Design review of the part built by this model. Coordinates are the model's own, in mm. Face numbers are marked on the shaded views. A direction names the side the tool comes from. Round coordinates to 2 decimals unless told otherwise and drop trailing zeros. Loops run counter-clockwise (first coordinate to the right, second up) from the corner with the lowest first, then second, coordinate; pieces in that order, holes last. Notation, with made-up numbers: (25, 48.5) -> (77, 48.5) arc R33 cw to (77, 79.5) -> close; hole circle Ø5 at (0, 40.25). An arc over 180 degrees is marked (long way). Answer as CSV lines item,"result". Start each with the question number.
(1) Take a section at C-C, the plane y = -3.25. Write out the cut boundary in (x, z), and give its area (3 significant figures).
(2) Draft analysis for pull direction Y (two halves, no side actions). For the marked faces 5, 6, 7 and 8, state which applies: +Y half, -Y half, draft (parallel to the pull), parting line (faces both ways), or undercut.
(3) Take a section at A-A, the plane x = 0. Write out the cut boundary in (y, z).
(4) Take a section at D-D, the plane x = -3.25. Write out the cut boundary in (y, z).
(5) Take a section at B-B, the plane z = 8.5. Write out the cut boundary in (x, y), and give its area (3 significant figures).
(6) Machinability: for the marked faces 1, 2, 3 and 4, which of the approach directions +Z, -Z, +X, -X, +Y, -Y give a long, thin tool a straight path to every point of the face, cutting with its end or side? Answer none if there is none.
(7) For P1, Ø1, axis at x = 6, z = 9.5, coming from the +Y side; P2, Ø0.6, axis at y = 8.5, z = 1.5, coming from the +X side; P3, Ø0.6, axis at y = 8.5, z = 1, coming from the -X side, all flat-tipped, find the tip position at first contact; note any pin that passes through.
(8) To check wall thickness, follow line 1 (Y direction, x = 0, z = 1.1); line 2 (Y direction, x = 0, z = 0.65); line 3 (Z direction, x = 1.5, y = -1.25). State the ranges of each line that lie inside material, in increasing order. Write a range as from..to.
from build123d import *

# Parameters (mm, degrees)
SKETCH1_W           = 20
SKETCH1_H           = 14
BOSS_EXTRUDE1_DEPTH = 12
SKETCH2_R           = 1.5
BOSS_EXTRUDE2_DEPTH = 2
SHELL2_START        = -6
SHELL2_OUTLINE_W    = 20
SHELL2_OUTLINE_H    = 10
SHELL2_DEPTH        = 12


# Read off the part's stored shape, not the designer's step: Shell2
with BuildPart() as part:
    # Sketch1 → Boss-Extrude1 (new body)
    with BuildSketch(Plane.XY):
        Rectangle(SKETCH1_W, SKETCH1_H)
    extrude(amount=BOSS_EXTRUDE1_DEPTH)

    # Sketch2 → Boss-Extrude2 (add)
    # profile 1 of 2: a face of its own
    with BuildSketch(Plane.XY):
        with BuildLine():
            Line((2.5, -9.5), (2.5, -7))
            Line((2.5, -7), (-2.5, -7))
            Line((-2.5, -7), (-2.5, -9.5))
            ThreePointArc((-2.5, -9.5), (0, -12), (2.5, -9.5))
        make_face()
        with Locations((0, -9.5)):
            Circle(SKETCH2_R, mode=Mode.SUBTRACT)
    # profile 2 of 2: a face of its own
    with BuildSketch(Plane.XY):
        with BuildLine():
            Line((2.5, 9.5), (2.5, 7))
            Line((2.5, 7), (-2.5, 7))
            Line((-2.5, 7), (-2.5, 9.5))
            ThreePointArc((-2.5, 9.5), (0, 12), (2.5, 9.5))
        make_face()
        with Locations((0, 9.5)):
            Circle(SKETCH2_R, mode=Mode.SUBTRACT)
    extrude(amount=BOSS_EXTRUDE2_DEPTH)

    # Shell2 outline → Shell2 (cut)
    with BuildSketch(Plane(origin=(0, 0, 0), x_dir=(1, 0, 0), z_dir=(0, 1, 0)).offset(SHELL2_START)):
        with Locations((0, -6)):
            Rectangle(SHELL2_OUTLINE_W, SHELL2_OUTLINE_H)
    extrude(amount=SHELL2_DEPTH, mode=Mode.SUBTRACT)


solid = part.part
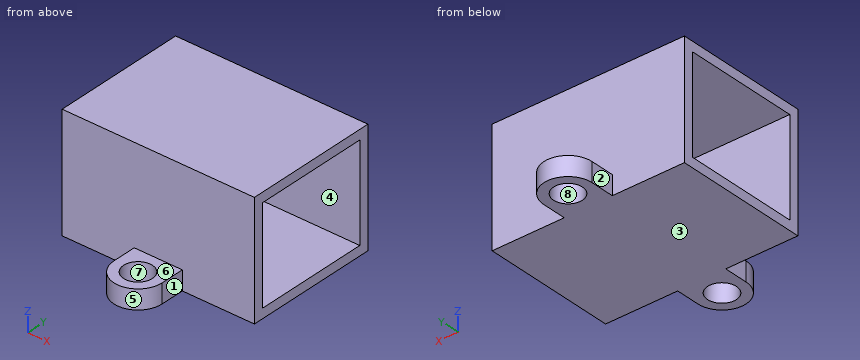
The answers:
1,outline,"(-10, 0) -> (10, 0) -> (10, 1) -> (-10, 1) -> close; (-10, 11) -> (10, 11) -> (10, 12) -> (-10, 12) -> close"
1,area,"40.0 mm²"
2,face 5,"-Y half"
2,face 6,"draft"
2,face 7,"undercut"
2,face 8,"undercut"
3,outline,"(-12, 0) -> (-11, 0) -> (-11, 2) -> (-12, 2) -> close; (-8, 0) -> (8, 0) -> (8, 2) -> (7, 2) -> (7, 12) -> (-7, 12) -> (-7, 2) -> (-8, 2) -> close; (11, 0) -> (12, 0) -> (12, 2) -> (11, 2) -> close; hole (-6, 1) -> (6, 1) -> (6, 11) -> (-6, 11) -> close"
4,outline,"(-7, 0) -> (7, 0) -> (7, 12) -> (-7, 12) -> close; hole (-6, 1) -> (6, 1) -> (6, 11) -> (-6, 11) -> close"
5,outline,"(-10, -7) -> (10, -7) -> (10, -6) -> (-10, -6) -> close; (-10, 6) -> (10, 6) -> (10, 7) -> (-10, 7) -> close"
5,area,"40.0 mm²"
6,face 1,"+Z, -Z, +X, -Y"
6,face 2,"+Z, -Z, -X, +Y"
6,face 3,"-Z, +X, -X, +Y, -Y"
6,face 4,"+X, -X"
7,P1,"y = 7"
7,P2,"x = 2.5"
7,P3,"x = -2.5"
8,line 1,"-12..-11, -8..-6, 6..8, 11..12"
8,line 2,"-12..-11, -8..8, 11..12"
8,line 3,"0..1, 11..12"
